from build123d import *

# Parameters (mm, degrees)
SKETCH2_W                = 35.2
SKETCH2_H                = 35.2
CUT_EXTRUDE1_DEPTH       = 4
SKETCH4_W                = 5.866666667
SKETCH4_H                = 3
SKETCH4_W_2              = 5.866666666
BOSS_EXTRUDE1_DEPTH      = 10
BOSS_EXTRUDE1_DEPTH_BACK = 63.5
SKETCH5_R                = 1.65
CUT_EXTRUDE2_DEPTH       = 11
SKETCH8_W                = 5.866666667
SKETCH8_H                = 3
SKETCH8_W_2              = 5.866666666
BOSS_EXTRUDE3_DEPTH      = 8


with BuildPart() as part:
    # Sketch1 → Revolve1 (revolve)
    with BuildSketch(Plane.XY):
        Polygon((0, 0), (63, 0), (69, 10), (65.501428863, 10), (61.301428863, 3), (0, 3), align=None)
    revolve(axis=Axis((0, 0, 0), (0, 1, 0)))

    # Sketch2 → Cut-Extrude1 (cut, through all)
    with BuildSketch(Plane(origin=(0, 3, 0), x_dir=(1, 0, 0), z_dir=(0, 1, 0))):
        with Locations((0, -36.1)):
            Rectangle(SKETCH2_W, SKETCH2_H)
    extrude(amount=-CUT_EXTRUDE1_DEPTH, mode=Mode.SUBTRACT)

    # Sketch4 → Boss-Extrude1 (add, two sides)
    with BuildSketch(Plane(origin=(0, 0, 0), x_dir=(0, 0, -1), z_dir=(1, 0, 0))) as boss_extrude1_sk:
        with Locations((-9.066666666, 4.5)):
            Rectangle(SKETCH4_W, SKETCH4_H)
        with Locations((0, 4.5)):
            Rectangle(SKETCH4_W_2, SKETCH4_H)
        with Locations((9.066666666, 4.5)):
            Rectangle(SKETCH4_W, SKETCH4_H)
    extrude(amount=BOSS_EXTRUDE1_DEPTH)
    extrude(boss_extrude1_sk.sketch, amount=-BOSS_EXTRUDE1_DEPTH_BACK)

    # Sketch5 → Cut-Extrude2 (cut, through all)
    with BuildSketch(Plane(origin=(0, 0, 0), x_dir=(1, 0, 0), z_dir=(0, 1, 0))):
        with Locations((7, -8.5)):
            Circle(SKETCH5_R)
        with Locations((7, 8.5)):
            Circle(SKETCH5_R)
        with Locations((-52, 8.5)):
            Circle(SKETCH5_R)
        with Locations((-52, -8.5)):
            Circle(SKETCH5_R)
    extrude(amount=CUT_EXTRUDE2_DEPTH, mode=Mode.SUBTRACT)

    # Sketch8 → Boss-Extrude3 (add)
    with BuildSketch(Plane(origin=(10, 0, 0), x_dir=(0, 0, -1), z_dir=(1, 0, 0))):
        with Locations((-9.066666666, 4.5)):
            Rectangle(SKETCH8_W, SKETCH8_H)
        with Locations((0, 4.5)):
            Rectangle(SKETCH8_W_2, SKETCH8_H)
        with Locations((9.066666666, 4.5)):
            Rectangle(SKETCH8_W, SKETCH8_H)
    extrude(amount=BOSS_EXTRUDE3_DEPTH)


solid = part.part
Build history of the part. All positions in model axes, mm. A direction names the side the tool comes from. Round coordinates to 2 decimals unless told otherwise and drop trailing zeros. Loops run counter-clockwise (first coordinate to the right, second up) from the corner with the lowest first, then second, coordinate; pieces in that order, holes last. Notation, with made-up numbers: (38.5, 43.5) -> (63.5, 43.5) arc R18 cw to (63.5, 55.5) -> close; hole circle Ø3 at (82.5, -7). An arc over 180 degrees is marked (long way). One line per item, written item: value. Start each with the question number.
Q1. Cut at A-A on x = 0. List the corners of the cut face in (y, z).
Q2. Drop flat-ended pins along their axis: pin 1 Ø1.5 at (x, y) = (3.5, 1) entering from -Z; pin 2 Ø6 at (y, z) = (5.5, -18.5) entering from +X; pin 3 Ø1.5 at (y, z) = (2, 42) entering from +X. Give the stop position or say it passes through.
Q3. Two-plate mould, pull along Z, no slides. Class faces 3 (the face through (-13.74, 0.63, 61.87)), 4 (the face through (-22, 6, 0)): released by +Z, released by -Z, zero draft, split by the parting line, or undercut.
Q4. Cut at B-B on z = 0. List the corners of the cut face in (x, y).
Q5. Probe line 1 along X through (y, z) = (4.6, 8.5); line 2 along X through (y, z) = (1.45, 8.5); line 3 along X through (y, z) = (3.35, 8.5). List the from-to ranges inside material, lowest first.
Q6. Cut at C-C on x = -52. Count the separate pieces of the cut face and the enclosed holes in it, plus the area to 3 significant figures.
Q7. 3-axis set-ups, long thin cutter, end or side, ignore diameter. For faces 1 (the face through (0, 2, 18.5)), 2 (the face through (-23, 4, 6.133)): which of +Z, -Z, +X, -X, +Y, -Y reach the whole face in a straight line?
Computed:
1. outline: (0, -63) -> (10, -69) -> (10, -65.5) -> (3, -61.3) -> (3, -12) -> (6, -12) -> (6, -6.13) -> (3, -6.13) -> (3, -2.93) -> (6, -2.93) -> (6, 2.93) -> (3, 2.93) -> (3, 6.13) -> (6, 6.13) -> (6, 12) -> (3, 12) -> (3, 18.5) -> (0, 18.5) -> close; (0, 53.7) -> (3, 53.7) -> (3, 61.3) -> (10, 65.5) -> (10, 69) -> (0, 63) -> close
2. pin 1: z = -63.96
2. pin 2: x = 65.71
2. pin 3: x = 49.43
3. face 3: split by the parting line
3. face 4: undercut
4. outline: (-69, 10) -> (-63, 0) -> (63, 0) -> (69, 10) -> (65.5, 10) -> (61.3, 3) -> (18, 3) -> (18, 6) -> (-63.1, 6) -> (-65.5, 10) -> close
5. line 1: -65.21 to -53.65, -50.35 to 5.35, 8.65 to 18, 61.68 to 65.21
5. line 2: -63.3 to -53.65, -50.35 to 5.35, 8.65 to 63.3
5. line 3: -64.45 to -53.65, -50.35 to 5.35, 8.65 to 18, 60.92 to 64.45
6. separate pieces: 3
6. enclosed holes: 0
6. area: 318 mm²
7. face 1: +Y, -Y
7. face 2: +Y
